Read the model definition and answer for the solid it produces. Units are mm, in the model's axes. A direction names the side the tool comes from. Round coordinates to 2 decimals unless told otherwise and drop trailing zeros. Order: outer loops, then holes, each group sorted by start corner. A loop starts at its lowest first (then second) coordinate and runs counter-clockwise, first axis right, second up. Notation, with made-up numbers: M -10.75,43 L 29.25,43 A19 ccw 29.25,66 Z; hole C 79.5,32.5 d3. An arc over 180 degrees is marked long. Answer as CSV lines item,"result".
```python
from build123d import *

# Parameters (mm, degrees)
F1_DEPTH  = 3.7
F2_W      = 78
F2_H      = 2.3
F3_DEPTH  = 1.5
F2_H_2    = 5.9
F4_DEPTH  = 3.2
F2_R      = 3.5
F5_DEPTH  = 4
F6_R      = 1.4
F7_DEPTH  = 6.3
F8_R      = 1.4
F9_DEPTH  = 6.3
F10_SIZE  = 3.3
F11_SCALE = 1.1


with BuildPart() as f1:
    # F0 (on Top) → F1 (new body)
    with BuildSketch(Plane.XY):
        with BuildLine():
            ThreePointArc((38, -13.75), (24.25, 0), (38, 13.75))
            Line((38, 13.75), (-38, 13.75))
            ThreePointArc((-38, 13.75), (-28.2772817587, 9.7227182413), (-24.25, 0))
            ThreePointArc((-24.25, 0), (-28.2772817587, -9.7227182413), (-38, -13.75))
            Line((-38, -13.75), (38, -13.75))
        make_face()
        with BuildLine():
            ThreePointArc((-24.25, 0), (-28.2772817587, 9.7227182413), (-38, 13.75))
            Line((-38, 13.75), (-38, -13.75))
            ThreePointArc((-38, -13.75), (-28.2772817587, -9.7227182413), (-24.25, 0))
        make_face()
        with BuildLine():
            Line((-38, -13.75), (-38, 13.75))
            ThreePointArc((-38, 13.75), (-51.75, 0), (-38, -13.75))
        make_face()
        with BuildLine():
            Line((38, -13.75), (38, 13.75))
            ThreePointArc((38, 13.75), (24.25, 0), (38, -13.75))
        make_face()
        with BuildLine():
            ThreePointArc((51.75, 0), (47.7227182413, 9.7227182413), (38, 13.75))
            Line((38, 13.75), (38, -13.75))
            ThreePointArc((38, -13.75), (47.7227182413, -9.7227182413), (51.75, 0))
        make_face()
    extrude(amount=F1_DEPTH)

    # F2 (on face) → F3 (cut)
    with BuildSketch(Plane.XY.offset(3.7)):
        with Locations((0, 9.85)):
            Rectangle(F2_W, F2_H)
        with Locations((0, 1.65)):
            Rectangle(F2_W, F2_H)
        with Locations((0, -1.65)):
            Rectangle(F2_W, F2_H)
        with Locations((0, -9.85)):
            Rectangle(F2_W, F2_H)
    extrude(amount=-F3_DEPTH, mode=Mode.SUBTRACT)

    # F2 (on face) → F4 (cut)
    with BuildSketch(Plane.XY.offset(3.7)):
        with Locations((0, 5.75)):
            Rectangle(F2_W, F2_H_2)
        with Locations((0, -5.75)):
            Rectangle(F2_W, F2_H_2)
    extrude(amount=-F4_DEPTH, mode=Mode.SUBTRACT)

    # F2 (on face) → F5 (join)
    with BuildSketch(Plane.XY.offset(3.7)):
        with Locations((45.75, 0)):
            Circle(F2_R)
        with Locations((-45.75, 0)):
            Circle(F2_R)
    extrude(amount=F5_DEPTH)

    # F6 (on face) → F7 (cut)
    with BuildSketch(Plane.XY.offset(7.7)):
        with Locations((45.75, 0)):
            Circle(F6_R)
    extrude(amount=-F7_DEPTH, mode=Mode.SUBTRACT)

    # F8 (on face) → F9 (cut)
    with BuildSketch(Plane.XY.offset(7.7)):
        with Locations((-45.75, 0)):
            Circle(F8_R)
    extrude(amount=-F9_DEPTH, mode=Mode.SUBTRACT)

    # F10
    f10_edges = [f1.edges().sort_by_distance(p)[0] for p in [
        (0, 13.75, 0),
    ]]
    chamfer(f10_edges, length=F10_SIZE)


with BuildPart() as f1_1:
    # F11: moved
    add(f1.part.scale(F11_SCALE))


solid = f1_1.part
```
Item 1: Flat-ended cylindrical pins translate along their axes: pin 1 (2 mm diameter, centred on x = 13.5, z = 1.5, fed in from -Y) (3 decimals); pin 2 (0.6 mm diameter, centred on x = -16, z = 1.5, fed in from +Y) (3 decimals); pin 3 (8 mm diameter, centred on x = -34.5, y = 0, fed in from +Z); pin 4 (0.5 mm diameter, centred on x = -15, z = 3.5, fed in from -Y) (3 decimals). Find the tip coordinate at first contact, or state that the pin passes through.
Ans:
pin 1,"y = -13.995"
pin 2,"y = 13.295"
pin 3,"z = 4.07"
pin 4,"y = -15.125"
Item 2: Find the intervals of material crossed by probe 1 along Y at (x, z) = (-26, 2.5) (3 decimals); probe 2 along X at (y, z) = (6.5, 2.5); probe 3 along Y at (x, z) = (-49, 5.25), in increasing order. Write a range as [from, to].
Ans:
probe 1,"[-13.995, -12.1], [-0.55, 0.55], [12.1, 13.995]"
probe 2,"[-54.19, -42.9], [42.9, 54.19]"
probe 3,"[-3.61, -0.78], [0.78, 3.61]"
Item 3: A cutting plane is placed at A-A, the plane z = 6.25. Determine the outline of the cut face in (x, y) (3 decimals), and give its area (3 significant figures).
Ans:
outline,"C -50.325,0 d7.7; C 50.325,0 d7.7; hole C -50.325,0 d3.08; hole C 50.325,0 d3.08"
area,"78.2 mm2"
Item 4: Determine the mould class of faces 3 (the face through (-50, -2, 8.47)), 4 (the face through (-53.47, 0.26, 0.18)), 5 (the face through (-1, 6, 0.55)) for opening direction X: +X half, -X half, draft (parallel to the pull), parting line (faces both ways), or undercut.
Ans:
face 3,"draft"
face 4,"-X half"
face 5,"undercut"
Item 5: A cutting plane is placed at B-B, the plane x = 26. Determine the outline of the cut face in (y, z) (3 decimals), and give its area (3 significant figures).
Ans:
outline,"M -15.125,3.63 L -11.495,0 L 11.495,0 L 15.125,3.63 L 15.125,4.07 L 12.1,4.07 L 12.1,2.42 L 9.57,2.42 L 9.57,0.55 L 3.08,0.55 L 3.08,2.42 L 0.55,2.42 L 0.55,4.07 L -0.55,4.07 L -0.55,2.42 L -3.08,2.42 L -3.08,0.55 L -9.57,0.55 L -9.57,2.42 L -12.1,2.42 L -12.1,4.07 L -15.125,4.07 Z"
area,"47.6 mm2"
Item 6: A tool of negligible diameter and unlimited length cuts with its end or side. For faces 1 (the face through (0.585, 13.285, 1.79)), 2 (the face through (-48.902, -0.59, 5.054)), from which of +Z, -Z, +X, -X, +Y, -Y can it reach the whole face along a straight path? Write none if from no direction.
Ans:
face 1,"-Z, +X, -X, +Y"
face 2,"+Z"
